Source: three-view drawing plus pictorial views. Frame: mm from the lowest corner of the part. A direction names the side the tool comes from. Coordinates: 2 decimals unless noted, no trailing zeros. Loops run counter-clockwise (first coordinate to the right, second up) from the corner with the lowest first, then second, coordinate; pieces in that order, holes last. Notation, with made-up numbers: M 10.25,50.5 L 17.25,50.5 A14 ccw 17.25,61.5 Z; hole C -16,-13.75 d11. An arc over 180 degrees is marked long. Use a Markdown table: item, result. Add a question column.
1. Set-up query: the marked faces 5, 6 and 7. Return all of +Z, -Z, +X, -X, +Y, -Y with unobstructed straight access to the full face (end or side cutting, diameter ignored); none if empty.
2. Line query: L1, parallel to X at y = 13.5, z = 1.45; L2, parallel to Y at x = 4.5, z = 0.95 (3 decimals). Output: solid intervals per line, ascending. Write a range as [from, to].
3. Section C-C on x = 11. Output: boundary loops of the cut face in (y, z).
4. Section B-B on y = 2.75. Output: boundary loops of the cut face in (x, z) (3 decimals), then the cut area to 3 significant figures.
5. Draft query along Y for the marked faces 1, 2, 3 and 4. Return one class per face: +Y half, -Y half, draft (parallel to the pull), parting line (faces both ways), or undercut.
6. Section A-A on z = 0.9. Output: boundary loops of the cut face in (x, y) (3 decimals).
7. Section D-D on y = 16.25. Output: boundary loops of the cut face in (x, z).
8. Pin query (flat end, axial travel): pin 1 (0.9 mm diameter, centred on y = 7, z = 1, fed in from -X). Return the tip coordinate at first contact, or that it passes through.
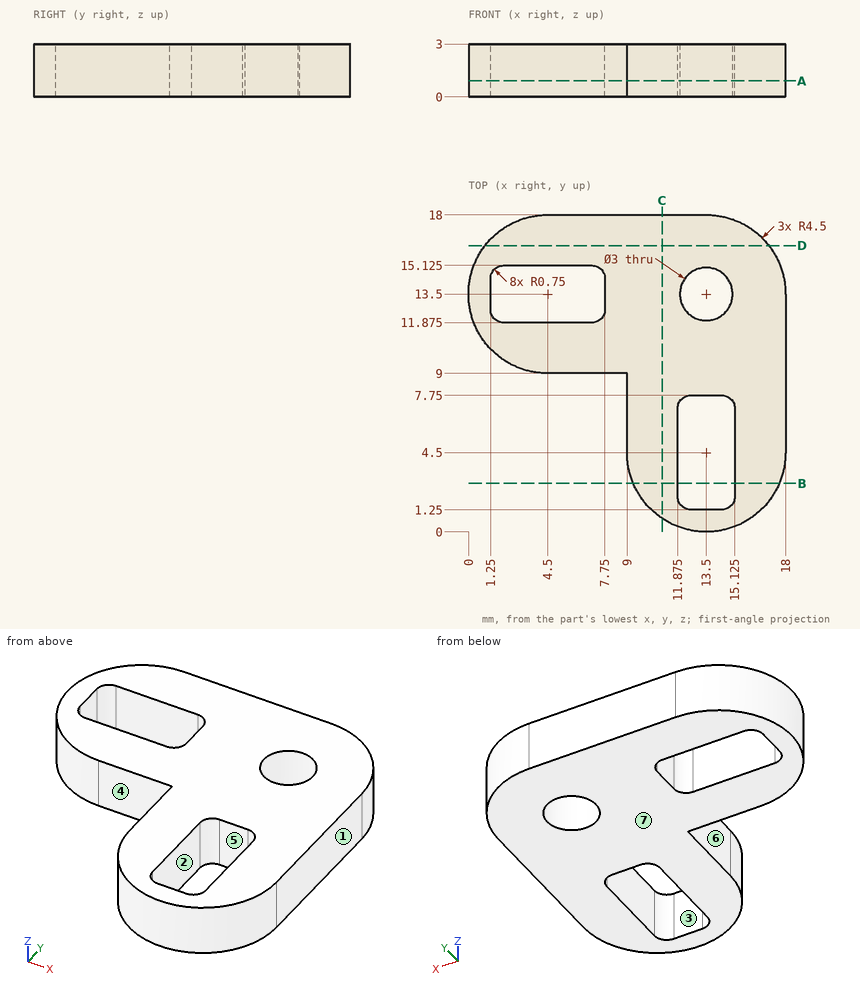
Answers below:
| question | item | result |
|---|---|---|
| 1 | face 5 | +Z, -Z |
| 1 | face 6 | +Z, -Z, -X, -Y |
| 1 | face 7 | -Z, +X, -X, +Y, -Y |
| 2 | L1 | x = [0, 1.25], [7.75, 12], [15, 18] |
| 2 | L2 | y = [9, 11.875], [15.125, 18] |
| 3 | outline | M 0.76,0 L 18,0 L 18,3 L 0.76,3 Z |
| 4 | outline | M 9.354,0 L 11.875,0 L 11.875,3 L 9.354,3 Z; M 15.125,0 L 17.646,0 L 17.646,3 L 15.125,3 Z |
| 4 | area | 15.1 mm² |
| 5 | face 1 | draft |
| 5 | face 2 | undercut |
| 5 | face 3 | undercut |
| 5 | face 4 | -Y half |
| 6 | outline | M 4.5,9 L 9,9 L 9,4.5 A4.5 ccw 18,4.5 L 18,13.5 A4.5 ccw 13.5,18 L 4.5,18 A4.5 ccw Z; hole M 1.25,12.625 A0.75 ccw 2,11.875 L 7,11.875 A0.75 ccw 7.75,12.625 L 7.75,14.375 A0.75 ccw 7,15.125 L 2,15.125 A0.75 ccw 1.25,14.375 Z; hole M 11.875,2 A0.75 ccw 12.625,1.25 L 14.375,1.25 A0.75 ccw 15.125,2 L 15.125,7 A0.75 ccw 14.375,7.75 L 12.625,7.75 A0.75 ccw 11.875,7 Z; hole C 13.5,13.5 d3 |
| 7 | outline | M 0.94,0 L 17.06,0 L 17.06,3 L 0.94,3 Z |
| 8 | pin 1 | stops at x = 9 |
